```python
from build123d import *

# Parameters (mm, degrees)
SKETCH3_R           = 35
BOSS_EXTRUDE1_DEPTH = 260
SKETCH4_R           = 20
CUT_EXTRUDE1_DEPTH  = 271


with BuildPart() as part:
    # Sketch1 → Revolve2 (revolve)
    with BuildSketch(Plane.XY):
        Polygon((0, 135), (0, -135), (50, -135), (50, -115), (30, -115), (30, 135), align=None)
    revolve(axis=Axis((0, 135, 0), (0, -1, 0)))

    # Sketch3 → Boss-Extrude1 (add)
    with BuildSketch(Plane(origin=(0, 0, 0), x_dir=(0, 0, 1), z_dir=(0.984807753, 0.173648178, 0))):
        with Locations((0, -32.949046657)):
            Circle(SKETCH3_R)
    extrude(amount=BOSS_EXTRUDE1_DEPTH)

    # Sketch4 → Cut-Extrude1 (cut, through all)
    with BuildSketch(Plane(origin=(0, 135, 0), x_dir=(1, 0, 0), z_dir=(0, 1, 0))):
        Circle(SKETCH4_R)
    extrude(amount=-CUT_EXTRUDE1_DEPTH, mode=Mode.SUBTRACT)


solid = part.part
```
Build history of the part. All positions in model axes, mm. A direction names the side the tool comes from. Give positions to 0.01 mm unless a question says otherwise; leave off trailing zeros. Loops run counter-clockwise (first coordinate to the right, second up) from the corner with the lowest first, then second, coordinate; pieces in that order, holes last. Notation, with made-up numbers: (5, 64.25) -> (63, 64.25) arc R22 ccw to (63, 101.25) -> close; hole circle Ø1 at (8.5, -2.5). An arc over 180 degrees is marked (long way). One line per question, with ' | ' between items. Start each with the question number.
1) Cut at B-B (z = -40). Give the cut face in (x, y).
2) 3-axis set-ups, long thin cutter, end or side, ignore diameter. For faces 4 (the flat face through (6, 135, -20)), 5 (the flat face through (22, -115, -22)), 6 (the flat face through (-5.853, 33.192, -31.816)), 7 (the flat face through (-5.853, 33.192, 31.726)), 8 (the cylindrical face through (47.69, -124.86, 15.02)): which of +Z, -Z, +X, -X, +Y, -Y reach the whole face in a straight line?
3) Pin check, flat tips, straight feed: pin 1 (1 mm diameter, centred on y = -60, z = -21.5, fed in from -X); pin 2 (1.5 mm diameter, centred on x = 180.5, z = -9.5, fed in from -Y); pin 3 (12 mm diameter, centred on x = 80, y = 82.5, fed in from -Z). Stop position of each tip, or through.
4) Probe L1, parallel to Z at x = 0, y = 14; L2, parallel to Y at x = 31, z = 4; L3, parallel to X at y = 53.5, z = 0.5. List the from-to ranges inside material, lowest first.
5) Cut at A-A (z = -3.5). Give the cut face in (x, y).
6) Two-plate mould, pull along Z, no slides. Class faces 1 (the flat face through (250.414, 77.114, -0.49)), 2 (the cylindrical face through (-29.97, 11.75, 1.32)), 3 (the cylindrical face through (-4.336, 1.89, 19.524)): released by +Z, released by -Z, zero draft, split by the parting line, or undercut.
Return value:
1) outline: (-30, -135) -> (30, -135) -> (30, -115) -> (-30, -115) -> close
2) face 4: +Z, -Z, +X, -X, +Y | face 5: none | face 6: -Z, -X | face 7: +Z, -X | face 8: -Y
3) pin 1: x = -21.42 | pin 2: y = 30.83 | pin 3: z = -20.45
4) L1: -30 to -20, 20 to 30 | L2: -135 to -115, 3.62 to 74.23 | L3: -30 to -19.99, 19.99 to 254.58
5) outline: (-49.88, -135) -> (-19.69, -135) -> (-19.69, 135) -> (-29.8, 135) -> (-29.8, -115) -> (-49.88, -115) -> close; (19.69, -135) -> (49.88, -135) -> (49.88, -115) -> (29.8, -115) -> (29.8, 3.35) -> (256.38, 43.3) -> (244.28, 111.89) -> (29.8, 74.07) -> (29.8, 135) -> (19.69, 135) -> close
6) face 1: zero draft | face 2: split by the parting line | face 3: undercut
